from build123d import *


with BuildPart() as part:
    # Sketch2 → Revolve1 (revolve)
    with BuildSketch(Plane.YZ, mode=Mode.PRIVATE) as revolve1_sk:
        with BuildLine():
            Line((-15, 0), (-9.864137891, 0))
            Line((-9.864137891, 0), (-7.663490214, -4.31901425))
            ThreePointArc((-7.663490214, -4.31901425), (-9.463525492, -6.426584774), (-9.68098575, -3.663490214))
            Line((-9.68098575, -3.663490214), (-10.783339073, -1.5))
            Line((-10.783339073, -1.5), (-13.5, -1.5))
            Line((-13.5, -1.5), (-13.5, -6.5))
            Line((-13.5, -6.5), (-15, -6.5))
            Line((-15, -6.5), (-15, 0))
        make_face()
    revolve(revolve1_sk.sketch.rotate(Axis((0, 0, 0), (0, 0, 1)), 270), axis=Axis((0, 0, 0), (0, 0, 1)))


solid = part.part
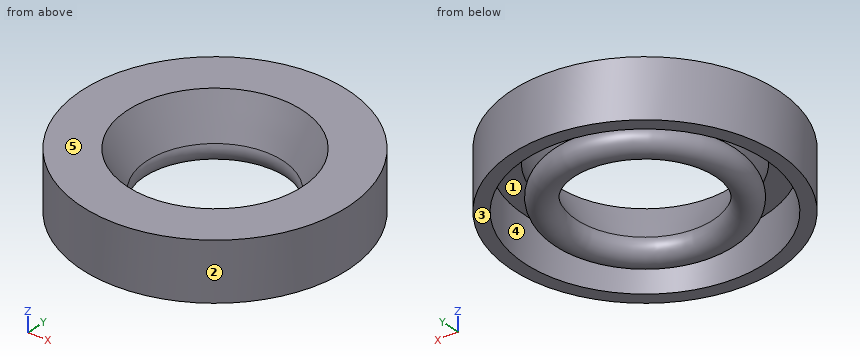
Could you check a few things on this model? Use its own coordinates, in mm. Face numbers are marked on the shaded views. A direction names the side the tool comes from. Coordinates: 2 decimals unless noted, no trailing zeros. Loops run counter-clockwise (first coordinate to the right, second up) from the corner with the lowest first, then second, coordinate; pieces in that order, holes last. Notation, with made-up numbers: (27.5, 3) -> (81.5, 3) arc R15 ccw to (81.5, 21) -> close; hole circle Ø1 at (40, 3.5). An arc over 180 degrees is marked (long way). Answer in a Markdown table with one row per item.
(1) Imagine slicing it at A-A (y = 0). List the corners of the cut face in (x, z) for me.
Results found:
| item | result |
|---|---|
| outline | (-15, -6.5) -> (-13.5, -6.5) -> (-13.5, -1.5) -> (-10.78, -1.5) -> (-9.68, -3.66) arc R1.5 ccw (long way) to (-7.66, -4.32) -> (-9.86, 0) -> (-15, 0) -> close; (7.66, -4.32) arc R1.5 ccw (long way) to (9.68, -3.66) -> (10.78, -1.5) -> (13.5, -1.5) -> (13.5, -6.5) -> (15, -6.5) -> (15, 0) -> (9.86, 0) -> close |
(2) Will this pin go through, and if not, where does the flat tip stop? pin 1 Ø2 at (x, y) = (10, 11.5) entering from +Z.
Results found:
| item | result |
|---|---|
| pin 1 | stops at z = 0 |
(3) If I drill on probe 1 along Y at (x, z) = (5.75, -5.5); probe 2 along X at (y, z) = (-2.5, -2.75); probe 3 along X at (y, z) = (-3.5, -4.5), over which ranges is the centre line in solid material (lowest first)?
Results found:
| item | result |
|---|---|
| probe 1 | y = -13.85 to -12.21, -8.68 to -4.95, 4.95 to 8.68, 12.21 to 13.85 |
| probe 2 | x = -14.79 to -13.27, -9.83 to -8.09, 8.09 to 9.83, 13.27 to 14.79 |
| probe 3 | x = -14.59 to -13.04, -9.81 to -6.73, 6.73 to 9.81, 13.04 to 14.59 |
(4) For the marked faces 4 and 5, which set-ups out of +Z, -Z, +X, -X, +Y, -Y let a thin tool reach every point of the face, with its end or its side?
Results found:
| item | result |
|---|---|
| face 4 | -Z |
| face 5 | +Z, +X, -X, +Y, -Y |
(5) Thinking about a two-plate mould opening in Y: for the marked faces 1, 2 and 3, which applies, released by +Y, released by -Y, zero draft, split by the parting line, or undercut?
Results found:
| item | result |
|---|---|
| face 1 | undercut |
| face 2 | split by the parting line |
| face 3 | zero draft |
